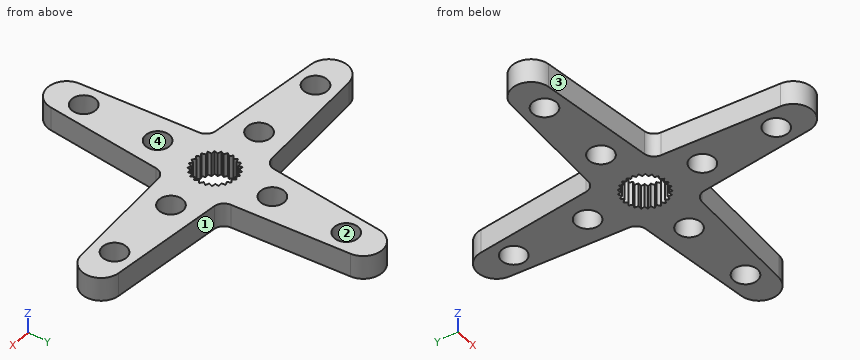
```python
from build123d import *

# Parameters (mm, degrees)
F0_R     = 1.6
F1_DEPTH = 3.175


# Not quite as in the source:
# - a length typed as a fraction of an inch, garbled in the dataset ("3 / 203.2 mm" for 3/8 in), is restored


with BuildPart() as f1:
    # F0 (on Top) → F1 (new body)
    with BuildSketch(Plane.XY):
        with BuildLine():
            ThreePointArc((-3.8043671626, 5.08), (-4.2086486587, 4.2104292787), (-5.08, 3.81))
            Line((-5.08, 3.81), (-20.32, 2.54))
            ThreePointArc((-20.32, 2.54), (-22.6579985335, 0), (-20.32, -2.54))
            Line((-20.32, -2.54), (-5.08, -3.8043671626))
            ThreePointArc((-5.08, -3.8043671626), (-4.2121628624, -4.2103745873), (-3.81, -5.08))
            Line((-3.81, -5.08), (-2.54, -20.32))
            ThreePointArc((-2.54, -20.32), (0, -22.6579985335), (2.54, -20.32))
            Line((2.54, -20.32), (3.8043671626, -5.08))
            ThreePointArc((3.8043671626, -5.08), (4.2103745873, -4.2121628624), (5.08, -3.81))
            Line((5.08, -3.81), (20.32, -2.54))
            ThreePointArc((20.32, -2.54), (22.6579985335, 0), (20.32, 2.54))
            Line((20.32, 2.54), (5.08, 3.8043671626))
            ThreePointArc((5.08, 3.8043671626), (4.2121628624, 4.2103745873), (3.81, 5.08))
            Line((3.81, 5.08), (2.54, 20.32))
            ThreePointArc((2.54, 20.32), (0, 22.6579985335), (-2.54, 20.32))
            Line((-2.54, 20.32), (-3.8043671626, 5.08))
        make_face()
        with Locations((-17.7799620532, -0.0219527348)):
            Circle(F0_R, mode=Mode.SUBTRACT)
        with Locations((-7.7799861494, 0)):
            Circle(F0_R, mode=Mode.SUBTRACT)
        with Locations((0.0219527348, -17.7799620532)):
            Circle(F0_R, mode=Mode.SUBTRACT)
        with Locations((0, -7.7799861494)):
            Circle(F0_R, mode=Mode.SUBTRACT)
        with Locations((7.7799861494, 0)):
            Circle(F0_R, mode=Mode.SUBTRACT)
        with Locations((-0.0219527348, 17.7799620532)):
            Circle(F0_R, mode=Mode.SUBTRACT)
        Polygon((-2.3131272616, 1.150841372), (-2.4811892868, 1.651717782), (-1.9542535042, 1.6899369317), (-1.992472654, 2.2168727143), (-1.4725868119, 2.1228475389), (-1.3785616365, 2.6427333809), (-0.8983920744, 2.4223718279), (-0.6780305213, 2.90254139), (-0.2677480588, 2.5696895861), (0.0651037451, 2.9799720486), (0.379719552, 2.555544297), (0.8041473037, 2.8701601039), (1.0033279869, 2.380824761), (1.4926633298, 2.5800054442), (1.5638936344, 2.0565092492), (2.0873898293, 2.1277395538), (2.0261940932, 1.6029756981), (2.5509579489, 1.5417799619), (2.3611813253, 1.0487212884), (2.8542399989, 0.8589446648), (2.547806851, 0.4285718633), (2.9781796525, 0.1221387154), (2.574344302, -0.2185063082), (2.9149893256, -0.6223416587), (2.4391262327, -0.8518549247), (2.6686394987, -1.3277180175), (2.1506488918, -1.4316783634), (2.2546092377, -1.9496689703), (1.7270383715, -1.9215441851), (1.6989135863, -2.4491150513), (1.1949116786, -2.2906723188), (1.0364689461, -2.7946742265), (0.5877042905, -2.5158690862), (0.3088991502, -2.9646337418), (-0.0564307197, -2.5829845462), (-0.4380799154, -2.9483144161), (-0.6970199802, -2.4878015876), (-1.1575328087, -2.7467416524), (-1.2938129119, -2.2363009057), (-1.8042536586, -2.3725810089), (-1.80931082, -1.8442852134), (-2.3376066155, -1.8493423749), (-2.2111230752, -1.3363862984), (-2.7240791517, -1.209902758), (-2.4740023355, -0.7445173173), (-2.9393877762, -0.4944405012), (-2.5814309304, -0.105867575), (-2.9700038565, 0.2520892708), (-2.5266587261, 0.5394342163), (-2.8140036716, 0.9827793468), align=None, mode=Mode.SUBTRACT)
        with Locations((0, 7.7799861494)):
            Circle(F0_R, mode=Mode.SUBTRACT)
        with Locations((17.7799620532, 0.0219527348)):
            Circle(F0_R, mode=Mode.SUBTRACT)
    extrude(amount=F1_DEPTH)


solid = f1.part
```
Work out the finished part from the listing and answer in its coordinate system (mm). Face numbers are marked on the shaded views. Give positions to 0.01 mm unless a question says otherwise; leave off trailing zeros. Loops run counter-clockwise (first coordinate to the right, second up) from the corner with the lowest first, then second, coordinate; pieces in that order, holes last. Notation, with made-up numbers: (37, 3) -> (91, 3) arc R28 cw to (91, 32) -> close; hole circle Ø9 at (58, 57.5). An arc over 180 degrees is marked (long way). Use CSV: the item, a comma, the result in double quotes.
1. The part is cut by section A-A (z = 2.25). State how many separate pieces and enclosed holes the cut face has, then the cut area to 3 significant figures.
Found:
separate pieces,"1"
enclosed holes,"9"
area,"433 mm^2"
2. The mould has two halves that part along Y. Classify the marked faces 1, 2, 3 and 4: +Y half, -Y half, draft (parallel to the pull), parting line (faces both ways), or undercut.
Found:
face 1,"+Y half"
face 2,"undercut"
face 3,"-Y half"
face 4,"undercut"
3. Straight lines are drawn through the part: line 1 (Y direction, x = -1, z = 1.65); line 2 (X direction, y = -1, z = 2.75); line 3 (X direction, y = -19, z = 0.65). For each, find the intervals that lie inside material, in ascending order.
Found:
line 1,"-22.45 to -19.01, -16.55 to -9.03, -6.53 to -2.66, 2.47 to 6.53, 9.03 to 16.51, 19.05 to 22.45"
line 2,"-22.45 to -19.05, -16.51 to -9.03, -6.53 to -2.61, 2.51 to 6.53, 9.03 to 16.55, 19.01 to 22.45"
line 3,"-2.65 to -1.01, 1.06 to 2.65"
4. The part is cut by section B-B (y = -12.5). Write down the section's boundary in (x, z) (3 decimals).
Found:
outline,"(-3.192, 0) -> (3.189, 0) -> (3.189, 3.175) -> (-3.192, 3.175) -> close"
5. The part is cut by section C-C (x = 15.5). Write down the section's boundary in (y, z) (3 decimals).
Found:
outline,"(-2.942, 0) -> (2.94, 0) -> (2.94, 3.175) -> (-2.942, 3.175) -> close"
